The listing builds one solid part. Answer for the finished solid, in the listing's coordinates (mm). A direction names the side the tool comes from. Round coordinates to 2 decimals unless told otherwise and drop trailing zeros. Order: outer loops, then holes, each group sorted by start corner. A loop starts at its lowest first (then second) coordinate and runs counter-clockwise, first axis right, second up. Notation, with made-up numbers: (11.5, 13) - (20.5, 13) arc R18 ccw to (20.5, 37) - close; hole circle Ø1 at (87.25, 82.25). An arc over 180 degrees is marked (long way). Use CSV: the item, a comma, the result in double quotes. Start each with the question number.
Item 1: Determine the mould class of faces 4 (the flat face through (23, 45, 2)), 5 (the flat face through (0, -45.846, 2)), 6 (the flat face through (-22.87, -37.1, 0.99)), 7 (the flat face through (20, -1, 2)) for opening direction X: +X half, -X half, draft (parallel to the pull), parting line (faces both ways), or undercut.
Item 2: Find section B-B, the plane x = 5.5. Give the vertices of the cut face in (y, z), plus the area to 3 significant figures.
Item 3: Find section A-A, the plane y = 8.5. Give the vertices of the cut face in (x, z).
Item 4: Straight lines are drawn through the part: line 1 along X through (y, z) = (-21.5, 1); line 2 along Y through (x, z) = (8, 1.8); line 3 along X through (y, z) = (-25.5, 0.9). For each, find the intervals that lie inside material, in ascending order. Write a range as [from, to].
Item 5: Flat-ended cylindrical pins translate along their axes: P1, Ø1.2, axis at x = -2, z = 1.5, coming from the -Y side; P2, Ø5, axis at x = -22.83, y = -41.82, coming from the +Z side; P3, Ø2, axis at y = 23, z = 2.5, coming from the +X side. Find the tip coordinate at first contact, or state that the pin passes through.
Item 6: For faces 1 (the flat face through (-25.83, -48, 1)), 2 (the flat face through (9.23, -13.33, 1.97)), 3 (the flat face through (0, -50, 2)), determine the directions among +Z, -Z, +X, -X, +Y, -Y from which every point of the face is accessible in a straight line to the end or side of a thin tool.
Item 7: Find section C-C, the plane x = 22.83. Give the vertices of the cut face in (y, z), plus the area to 3 significant figures.
```python
from build123d import *

# Parameters (mm, degrees)
F1_DEPTH = 4
F2_DEPTH = 2
F3_D     = 3
F4_R     = 1


with BuildPart() as f1:
    # F0 (on Top) → F1 (new body)
    with BuildSketch(Plane.XY):
        Polygon((20, 34.2358313501), (20, 50), (-20, 50), (-20, 34.2358313501), (-20, -34.2358313501), (-20, -50), (20, -50), (20, -34.2358313501), align=None)
        Polygon((16.206420958, -42.3818695248), (16.206420958, -45.8463579416), (13.757067936, -45.8463579416), (-13.757067936, -45.8463579416), (-16.206420958, -45.8463579416), (-16.206420958, -42.3818695248), (-16.206420958, -3.4644884169), (-16.206420958, -2), (-16.206420958, 0), (-16.206420958, 2), (-16.206420958, 3.4644884169), (-16.206420958, 42.3818695248), (-16.206420958, 45.8463579416), (-13.757067936, 45.8463579416), (13.757067936, 45.8463579416), (16.206420958, 45.8463579416), (16.206420958, 42.3818695248), (16.206420958, 3.4644884169), (16.206420958, 2), (16.206420958, 0), (16.206420958, -2), (16.206420958, -3.4644884169), align=None, mode=Mode.SUBTRACT)
        Polygon((1.224676511, 24.6554231792), (16.206420958, 45.8463579416), (13.757067936, 45.8463579416), (0, 26.3876673877), align=None)
        Polygon((2.4493530221, 22.9231789708), (16.206420958, 42.3818695248), (16.206420958, 45.8463579416), (1.224676511, 24.6554231792), align=None)
        Polygon((-2.4493530221, 22.9231789708), (-1.224676511, 24.6554231792), (-16.206420958, 45.8463579416), (-16.206420958, 42.3818695248), align=None)
        Polygon((-16.206420958, 45.8463579416), (-1.224676511, 24.6554231792), (0, 26.3876673877), (-13.757067936, 45.8463579416), align=None)
        Polygon((-16.206420958, -42.3818695248), (-16.206420958, -45.8463579416), (-1.224676511, -24.6554231792), (-2.4493530221, -22.9231789708), align=None)
        Polygon((-16.206420958, -45.8463579416), (-13.757067936, -45.8463579416), (0, -26.3876673877), (-1.224676511, -24.6554231792), align=None)
        Polygon((1.224676511, -24.6554231792), (16.206420958, -45.8463579416), (16.206420958, -42.3818695248), (2.4493530221, -22.9231789708), align=None)
        Polygon((13.757067936, -45.8463579416), (16.206420958, -45.8463579416), (1.224676511, -24.6554231792), (0, -26.3876673877), align=None)
        Polygon((14.7924442161, 2), (16.206420958, 2), (16.206420958, 3.4644884169), (2.4493530221, 22.9231789708), (1.224676511, 21.1909347624), align=None)
        Polygon((-16.206420958, 3.4644884169), (-16.206420958, 2), (-14.7924442161, 2), (-1.224676511, 21.1909347624), (-2.4493530221, 22.9231789708), align=None)
        Polygon((-2.4493530221, -22.9231789708), (-1.224676511, -21.1909347624), (-14.7924442161, -2), (-16.206420958, -2), (-16.206420958, -3.4644884169), align=None)
        Polygon((2.4493530221, -22.9231789708), (16.206420958, -3.4644884169), (16.206420958, -2), (14.7924442161, -2), (1.224676511, -21.1909347624), align=None)
        Polygon((12.343091194, 2), (14.7924442161, 2), (1.224676511, 21.1909347624), (0, 19.458690554), align=None)
        Polygon((-1.224676511, 21.1909347624), (-14.7924442161, 2), (-12.343091194, 2), (0, 19.458690554), align=None)
        Polygon((-14.7924442161, -2), (-1.224676511, -21.1909347624), (0, -19.458690554), (-12.343091194, -2), align=None)
        Polygon((0, -19.458690554), (1.224676511, -21.1909347624), (14.7924442161, -2), (12.343091194, -2), align=None)
        Polygon((14.7924442161, -2), (16.206420958, 0), (13.757067936, 0), (12.343091194, -2), align=None)
        Polygon((13.757067936, 0), (16.206420958, 0), (14.7924442161, 2), (12.343091194, 2), align=None)
        Polygon((-16.206420958, 0), (-14.7924442161, -2), (-12.343091194, -2), (-13.757067936, 0), align=None)
        Polygon((-14.7924442161, 2), (-16.206420958, 0), (-13.757067936, 0), (-12.343091194, 2), align=None)
        Polygon((0, 22.9231789708), (1.224676511, 21.1909347624), (2.4493530221, 22.9231789708), (1.224676511, 24.6554231792), align=None)
        Polygon((-1.224676511, 24.6554231792), (0, 22.9231789708), (1.224676511, 24.6554231792), (0, 26.3876673877), align=None)
        Polygon((-1.224676511, 21.1909347624), (0, 22.9231789708), (-1.224676511, 24.6554231792), (-2.4493530221, 22.9231789708), align=None)
        Polygon((0, 19.458690554), (1.224676511, 21.1909347624), (0, 22.9231789708), (-1.224676511, 21.1909347624), align=None)
        Polygon((-1.224676511, -21.1909347624), (0, -22.9231789708), (1.224676511, -21.1909347624), (0, -19.458690554), align=None)
        Polygon((0, -22.9231789708), (1.224676511, -24.6554231792), (2.4493530221, -22.9231789708), (1.224676511, -21.1909347624), align=None)
        Polygon((0, -26.3876673877), (1.224676511, -24.6554231792), (0, -22.9231789708), (-1.224676511, -24.6554231792), align=None)
        Polygon((-1.224676511, -24.6554231792), (0, -22.9231789708), (-1.224676511, -21.1909347624), (-2.4493530221, -22.9231789708), align=None)
        Polygon((14.7924442161, -2), (16.206420958, -2), (16.206420958, 0), align=None)
        Polygon((14.7924442161, 2), (16.206420958, 0), (16.206420958, 2), align=None)
        Polygon((-16.206420958, 2), (-16.206420958, 0), (-14.7924442161, 2), align=None)
        Polygon((-16.206420958, -2), (-14.7924442161, -2), (-16.206420958, 0), align=None)
    extrude(amount=F1_DEPTH)

    # F0 (on Top) → F2 (join)
    with BuildSketch(Plane.XY):
        Polygon((25.830000639, 55.8186091483), (20, 50), (20, 34.2358313501), (25.830000639, 40.0544404984), align=None)
        Polygon((-20, 34.2358313501), (-20, 50), (-25.830000639, 55.8186091483), (-25.830000639, 40.0544404984), align=None)
        Polygon((-20, -50), (-20, -34.2358313501), (-25.830000639, -40.0544404984), (-25.830000639, -55.8186091483), align=None)
        Polygon((25.830000639, -40.0544404984), (20, -34.2358313501), (20, -50), (25.830000639, -55.8186091483), align=None)
    extrude(amount=F2_DEPTH)

    # F3 (through all)
    with Locations(Plane(origin=(0, 0, 0), x_dir=(1, 0, 0), z_dir=(0, 0, -1))):
        with Locations((22.830000639, -48.6315488815), (22.830000639, -41.8172627687), (-22.830000639, -48.6315488815), (-22.830000639, -41.8172627687), (-22.830000639, 41.8172627687), (-22.830000639, 48.6315488815), (22.830000639, 41.8172627687), (22.830000639, 48.6315488815)):
            Hole(F3_D / 2)

    # F4
    f4_edges = [f1.edges().sort_by_distance(p)[0] for p in [
        (0, 50, 4),
        (0, 50, 0),
    ]]
    fillet(f4_edges, radius=F4_R)


solid = f1.part
```
Worked out:
1,face 4,"draft"
1,face 5,"undercut"
1,face 6,"-X half"
1,face 7,"+X half"
2,outline,"(-50, 0) - (-45.85, 0) - (-45.85, 4) - (-50, 4) - close; (-34.17, 0) - (-27.24, 0) - (-27.24, 4) - (-34.17, 4) - close; (-18.61, 0) - (-11.68, 0) - (-11.68, 4) - (-18.61, 4) - close; (11.68, 0) - (18.61, 0) - (18.61, 4) - (11.68, 4) - close; (27.24, 0) - (34.17, 0) - (34.17, 4) - (27.24, 4) - close; (45.85, 0) - (49, 0) arc R1 ccw to (50, 1) - (50, 3) arc R1 ccw to (49, 4) - (45.85, 4) - close"
2,area,"144 mm²"
3,outline,"(-20, 0) - (-16.21, 0) - (-16.21, 4) - (-20, 4) - close; (-12.65, 0) - (-7.75, 0) - (-7.75, 4) - (-12.65, 4) - close; (7.75, 0) - (12.65, 0) - (12.65, 4) - (7.75, 4) - close; (16.21, 0) - (20, 0) - (20, 4) - (16.21, 4) - close"
4,line 1,"x = [-20, -16.21], [-3.46, 3.46], [16.21, 20]"
4,line 2,"y = [-50, -45.85], [-37.7, -30.77], [-15.07, -8.14], [8.14, 15.07], [30.77, 37.7], [45.85, 50]"
4,line 3,"x = [-20, -16.21], [-4.27, 4.27], [16.21, 20]"
5,P1,"stops at y = -50"
5,P2,"stops at z = 2"
5,P3,"stops at x = 20"
6,face 1,"+Z, -Z, -X, +Y, -Y"
6,face 2,"+Z, -Z"
6,face 3,"+Z, -Z, -Y"
7,outline,"(-52.82, 0) - (-50.13, 0) - (-50.13, 2) - (-52.82, 2) - close; (-47.13, 0) - (-43.32, 0) - (-43.32, 2) - (-47.13, 2) - close; (-40.32, 0) - (-37.06, 0) - (-37.06, 2) - (-40.32, 2) - close; (37.06, 0) - (40.32, 0) - (40.32, 2) - (37.06, 2) - close; (43.32, 0) - (47.13, 0) - (47.13, 2) - (43.32, 2) - close; (50.13, 0) - (52.82, 0) - (52.82, 2) - (50.13, 2) - close"
7,area,"39.1 mm²"
